Input: part model. Units: mm. Frame: model coordinates. Give positions to 0.01 mm unless a question says otherwise; leave off trailing zeros. Order: outer loops, then holes, each group sorted by start corner. A loop starts at its lowest first (then second) coordinate and runs counter-clockwise, first axis right, second up. Notation, with made-up numbers: M 42.25,7 L 94.25,7 A28 cw 94.25,35 Z; hole C 59,46.25 d2. An arc over 180 degrees is marked long. Use a Markdown table: item, result.
from build123d import *

# Parameters (mm, degrees)
SKETCH3_W               = 25.4
SKETCH3_H               = 15.875
EXTRUDE2_DEPTH          = 125.73
F_1_4_CLEARANCE_HOLE1_D = 7.14248


with BuildPart() as part:
    # Sketch3 → Extrude2 (new, symmetric)
    with BuildSketch(Plane(origin=(0, 0, 0), x_dir=(0, 0, -1), z_dir=(1, 0, 0))):
        Rectangle(SKETCH3_W, SKETCH3_H)
    extrude(amount=EXTRUDE2_DEPTH, both=True)

    # 1/4 Clearance Hole1 (through all)
    with Locations(Plane(origin=(101.6, 7.9375, 0), x_dir=(0, 0, 1), z_dir=(0, 1, 0))):
        with Locations((0, 0), (0, -203.2)):
            Hole(F_1_4_CLEARANCE_HOLE1_D / 2)


solid = part.part
1) Material intervals for line 1 (X direction, y = 2.5, z = 0), sorted ascending. Write a range as from..to.
Response values:
| item | result |
|---|---|
| line 1 | x = -125.73..-105.17, -98.03..98.03, 105.17..125.73 |
2) Cut plane A-A on x = -101.6. Return loops of the section in (y, z), and give its area (3 significant figures).
Response values:
| item | result |
|---|---|
| outline | M -7.94,-12.7 L 7.94,-12.7 L 7.94,-3.57 L -7.94,-3.57 Z; M -7.94,3.57 L 7.94,3.57 L 7.94,12.7 L -7.94,12.7 Z |
| area | 290 mm² |
3) Mould query, pull axis X, two halves, no side actions, for faces 1 (the face through (-125.73, 0, 0)), 2 (the face through (2, 0, -12.7)), 3 (the face through (105.14, -0.11, 0.46)). Classes: released by +X, released by -X, zero draft, split by the parting line, or undercut.
Response values:
| item | result |
|---|---|
| face 1 | released by -X |
| face 2 | zero draft |
| face 3 | undercut |
4) Cut plane B-B on z = 0. Return loops of the section in (x, y).
Response values:
| item | result |
|---|---|
| outline | M -125.73,-7.94 L -105.17,-7.94 L -105.17,7.94 L -125.73,7.94 Z; M -98.03,-7.94 L 98.03,-7.94 L 98.03,7.94 L -98.03,7.94 Z; M 105.17,-7.94 L 125.73,-7.94 L 125.73,7.94 L 105.17,7.94 Z |
